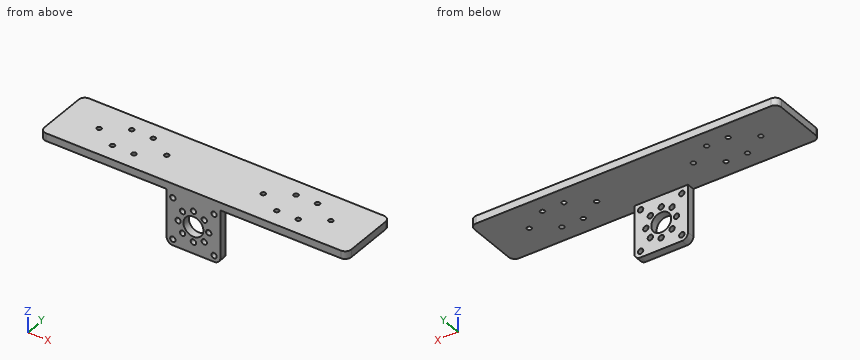
from build123d import *

# Parameters (mm, degrees)
ESQUISSE1_W             = 200
ESQUISSE1_H             = 40
BOSS_EXTRU_1_DEPTH      = 5
ESQUISSE5_W             = 35
ESQUISSE5_H             = 5
BOSS_EXTRU_3_DEPTH      = 35
ESQUISSE6_R             = 2.5
ENL_V_MAT_EXTRU_2_DEPTH = 35
ESQUISSE9_R             = 1.5
ENL_V_MAT_EXTRU_3_DEPTH = 35
CONG_2_R                = 4
ESQUISSE11_W            = 32.65685425
ESQUISSE11_H            = 33.828427125
BOSS_EXTRU_4_DEPTH      = 5
ESQUISSE14_R            = 6.5
ESQUISSE14_R_2          = 1.75
ESQUISSE14_R_3          = 1.749999999
ENL_V_MAT_EXTRU_4_DEPTH = 5


with BuildPart() as part:
    # Esquisse1 → Boss.-Extru.1 (new body)
    with BuildSketch(Plane.XY):
        with Locations((100, 20)):
            Rectangle(ESQUISSE1_W, ESQUISSE1_H)
    extrude(amount=-BOSS_EXTRU_1_DEPTH)

    # Esquisse5 → Boss.-Extru.3 (add)
    with BuildSketch(Plane(origin=(0, 0, -5), x_dir=(-1, 0, 0), z_dir=(0, 0, -1))):
        with Locations((-100, 2.5)):
            Rectangle(ESQUISSE5_W, ESQUISSE5_H)
    extrude(amount=BOSS_EXTRU_3_DEPTH)

    # Esquisse6 → Enlèv. mat.-Extru.2 (cut)
    with BuildSketch(Plane(origin=(0, 5, 0), x_dir=(1, 0, 0), z_dir=(0, 1, 0))):
        with Locations(Location((86.567832378, 36.000002876, 0), (0, 0, 270))):
            Circle(ESQUISSE6_R)
        with Locations(Location((113.567832366, 36.000575195, 0), (0, 0, 270))):
            Circle(ESQUISSE6_R)
        with Locations(Location((113.567832366, 9.000575195, 0), (0, 0, 270))):
            Circle(ESQUISSE6_R)
        with Locations(Location((86.5, 9.000575195, 0), (0, 0, 270))):
            Circle(ESQUISSE6_R)
    extrude(amount=-ENL_V_MAT_EXTRU_2_DEPTH, mode=Mode.SUBTRACT)

    # Esquisse9 → Enlèv. mat.-Extru.3 (cut)
    with BuildSketch(Plane.XY):
        with Locations((160.5, 11)):
            Circle(ESQUISSE9_R)
        with Locations((160.5, 29)):
            Circle(ESQUISSE9_R)
        with Locations((131.5, 20)):
            Circle(ESQUISSE9_R)
        with Locations(Location((68.5, 20, 0), (0, 0, 180))):
            Circle(ESQUISSE9_R)
        with Locations(Location((39.5, 29, 0), (0, 0, 180))):
            Circle(ESQUISSE9_R)
        with Locations(Location((39.5, 11, 0), (0, 0, 180))):
            Circle(ESQUISSE9_R)
        with Locations((24.5, 20)):
            Circle(ESQUISSE9_R)
        with Locations((53.5, 11)):
            Circle(ESQUISSE9_R)
        with Locations((53.5, 29)):
            Circle(ESQUISSE9_R)
        with Locations(Location((175.5, 20, 0), (0, 0, 180))):
            Circle(ESQUISSE9_R)
        with Locations(Location((146.5, 11, 0), (0, 0, 180))):
            Circle(ESQUISSE9_R)
        with Locations(Location((146.5, 29, 0), (0, 0, 180))):
            Circle(ESQUISSE9_R)
    extrude(amount=-ENL_V_MAT_EXTRU_3_DEPTH, mode=Mode.SUBTRACT)

    # Congé2
    cong_2_edges = [part.edges().sort_by_distance(p)[0] for p in [
        (117.5, 2.5, -40),
        (82.5, 2.5, -40),
        (0, 40, -2.5),
        (200, 40, -2.5),
        (200, 0, -2.5),
        (0, 0, -2.5),
    ]]
    fillet(cong_2_edges, radius=CONG_2_R)

    # Esquisse11 → Boss.-Extru.4 (add)
    with BuildSketch(Plane(origin=(0, 5, 0), x_dir=(1, 0, 0), z_dir=(0, 1, 0))):
        with Locations((100, 21.914213563)):
            Rectangle(ESQUISSE11_W, ESQUISSE11_H)
    extrude(amount=-BOSS_EXTRU_4_DEPTH)

    # Esquisse14 → Enlèv. mat.-Extru.4 (cut)
    with BuildSketch(Plane(origin=(0, 5, 0), x_dir=(1, 0, 0), z_dir=(0, 1, 0))):
        with Locations(Location((99.935028631, 22.564970946, 0), (0, 0, 270))):
            Circle(ESQUISSE14_R)
        with Locations(Location((99.935028631, 32.564970946, 0), (0, 0, 270))):
            Circle(ESQUISSE14_R_2)
        with Locations(Location((107.006096654, 29.636038546, 0), (0, 0, 270))):
            Circle(ESQUISSE14_R_2)
        with Locations(Location((109.935028631, 22.564970946, 0), (0, 0, 270))):
            Circle(ESQUISSE14_R_2)
        with Locations(Location((107.006096443, 15.493903134, 0), (0, 0, 270))):
            Circle(ESQUISSE14_R_2)
        with Locations(Location((99.935028631, 12.564970946, 0), (0, 0, 270))):
            Circle(ESQUISSE14_R_2)
        with Locations(Location((92.863960819, 15.493903134, 0), (0, 0, 270))):
            Circle(ESQUISSE14_R_2)
        with Locations(Location((89.935028631, 22.564970946, 0), (0, 0, 270))):
            Circle(ESQUISSE14_R_2)
        with Locations(Location((92.863961011, 29.636038989, 0), (0, 0, 270))):
            Circle(ESQUISSE14_R_3)
        with Locations(Location((113.370057685, 35.999999577, 0), (0, 0, 270))):
            Circle(ESQUISSE14_R_2)
        with Locations(Location((113.370057473, 9.129942103, 0), (0, 0, 270))):
            Circle(ESQUISSE14_R_2)
        with Locations(Location((86.5, 36, 0), (0, 0, 270))):
            Circle(ESQUISSE14_R_2)
        with Locations(Location((86.499999788, 9.129942103, 0), (0, 0, 270))):
            Circle(ESQUISSE14_R_2)
    extrude(amount=-ENL_V_MAT_EXTRU_4_DEPTH, mode=Mode.SUBTRACT)


solid = part.part
The listing builds one solid part. Answer for the finished solid, in the listing's coordinates (mm). Give positions to 0.01 mm unless a question says otherwise; leave off trailing zeros. Order: outer loops, then holes, each group sorted by start corner. A loop starts at its lowest first (then second) coordinate and runs counter-clockwise, first axis right, second up. Notation, with made-up numbers: (61, -1.5) - (94, -1.5) arc R17 cw to (94, 8.5) - close; hole circle Ø4 at (3, 16.25). An arc over 180 degrees is marked (long way). One line per item, written item: value. Start each with the question number.
1) Given pin 1 Ø6 at (x, y) = (121, 34) entering from +Z; pin 2 Ø4 at (x, y) = (152.5, 20.5) entering from -Z; pin 3 Ø2.5 at (y, z) = (1.5, -13) entering from -X; pin 4 Ø5.5 at (x, z) = (92.86, -29.64) entering from +Y, each flat-ended and moving along its own axis, determine where each tip first touches the part or whether it passes through.
2) A cutting plane is placed at B-B on y = 16. Give the vertices of the cut face in (x, z).
3) A cutting plane is placed at A-A on z = -22.5. Give the vertices of the cut face in (x, y), then the cut area to 3 significant figures.
4) A cutting plane is placed at C-C on x = 169. Give the vertices of the cut face in (y, z).
5) Find the intervals of material crossed by L1, parallel to Z at x = 100.5, y = 21.5, in increasing order.
Answer sheet:
1. pin 1: stops at z = 0
1. pin 2: stops at z = -5
1. pin 3: stops at x = 82.5
1. pin 4: stops at y = 5
2. outline: (0, -5) - (200, -5) - (200, 0) - (0, 0) - close
3. outline: (82.5, 0) - (88.19, 0) - (88.19, 5) - (82.5, 5) - close; (91.68, 0) - (93.44, 0) - (93.44, 5) - (91.68, 5) - close; (106.43, 0) - (108.19, 0) - (108.19, 5) - (106.43, 5) - close; (111.68, 0) - (117.5, 0) - (117.5, 5) - (111.68, 5) - close
3. area: 75.0 mm2
4. outline: (0, -5) - (40, -5) - (40, 0) - (0, 0) - close
5. L1: z = -5 to 0
